Autodesk Inventor part; units mm, degrees
ref_plane "YZ Plane" through (0, 0, 0) normal (1, 0, 0) x (0, 1, 0)
ref_plane "XZ Plane" through (0, 0, 0) normal (0, 1, 0) x (-1, 0, 0)
ref_plane "XY Plane" through (0, 0, 0) normal (0, 0, 1) x (1, 0, 0)
sketch "Sketch1" plane through (0, 0, 0) normal (0, 1, 0) x (-1, 0, 0)
  line L0 (0, 0) -> (-37, 0)
  line L1 (-37, 0) -> (-37, 37)
  line L2 (-37, 37) -> (0, 37)
  line L3 (0, 37) -> (0, 0)
  circle A0 centre (-18.5, 18.5) radius 15.5
  point P0 (-18.5, 0)
  dimension "d0" = 37
  dimension "d1" = 37
  dimension "d2" = 18.5
  dimension "d3" = 18.5
  dimension "d4" = 31
extrude "Extrusion1" add sketch "Sketch1" against normal blind 35
sketch "Sketch3" plane through (0, 0, 37) normal (0, 0, 1) x (1, 0, 0)
  circle A0 centre (18.5, -10) radius 4.5
  line L0 (37, 0) -> (37, -35)
  point P0 (0, 0)
  dimension "d8" = 9
  dimension "d18" = 18.5
extrude "Extrusion2" cut sketch "Sketch3" against normal blind 5
sketch "Sketch4" plane through (37, 0, 0) normal (0, 0, -1) x (-1, 0, 0)
  circle A0 centre (18.5, -10) radius 4.5
  circle A1 centre (18.5, -10) radius 2.5
  point P0 (37, 0)
  dimension "d11" = 5
extrude "Extrusion3" cut sketch "Sketch4" against normal blind 5 contours A1
sketch "Sketch5" plane through (0, 0, 37) normal (0, 0, 1) x (1, 0, 0)
  line L0 (37, 0) -> (0, 0)
  line L1 (0, -35) -> (37, -35)
  line L2 (0, 0) -> (37, 0)
  line L3 (37, 0) -> (37, -35)
  line L4 (37, -35) -> (0, -35)
  line L5 (0, -35) -> (0, 0)
  line L6 (0, 0) -> (0, -35)
  line L7 (0, 0) -> (37, 0)
  line L8 (37, 0) -> (37, -35)
  line L9 (37, -35) -> (0, -35)
  line L10 (0, -35) -> (0, 0)
  circle A0 centre (18.5, -25) radius 4.5
  dimension "d19" = 18.5
  dimension "d22" = 10
extrude "Extrusion4" add sketch "Sketch5" along normal blind 2
sketch "Sketch6" plane through (0, 0, 39) normal (0, 0, 1) x (1, 0, 0)
  line L0 (0, 0) -> (0, -35)
  line L1 (0, -35) -> (37, -35)
  line L2 (0, 0) -> (37, 0)
  line L3 (37, 0) -> (37, -35)
  line L4 (37, -35) -> (0, -35)
  line L5 (0, -35) -> (0, 0)
extrude "Extrusion5" add sketch "Sketch6" along normal blind 5
sketch "Sketch7" plane through (0, 0, 44) normal (0, 0, 1) x (1, 0, 0)
  circle A0 centre (18.5, -10) radius 2.5
  line L0 (37, 0) -> (0, 0)
  line L1 (37, -35) -> (37, 0)
  point P0 (18.5, 0)
  dimension "d24" = 5
  dimension "d25" = 10
  dimension "d26" = 18.5
extrude "Extrusion6" cut sketch "Sketch7" against normal through all
equation "\"d0\" = d1"
properties part number "welco mount v03b"
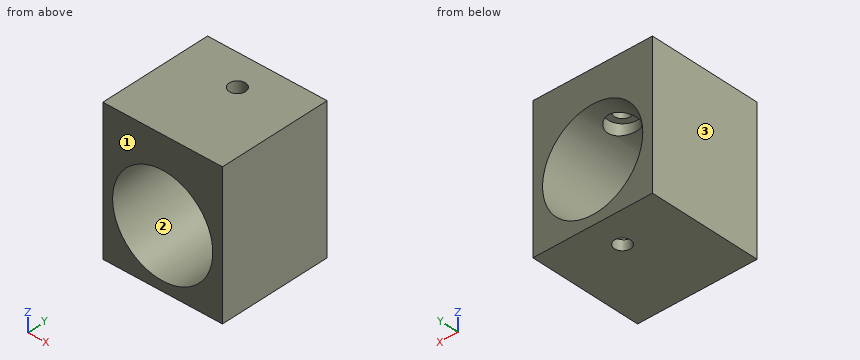
CAD build for the part. Positions are in the model's coordinates, mm. Face numbers are marked on the shaded views. Coordinates: 2 decimals unless noted, no trailing zeros. Loops run counter-clockwise (first coordinate to the right, second up) from the corner with the lowest first, then second, coordinate; pieces in that order, holes last. Notation, with made-up numbers: (19, -7.5) - (26, -7.5) arc R26 cw to (26, 7.5) - close; hole circle Ø9 at (-38, -13). An arc over 180 degrees is marked (long way). Use CSV: the item, a comma, the result in double quotes. Start each with the question number.
Q1. Cut at D-D, the plane x = 31.5. List the corners of the cut face in (y, z), then the cut area to 3 significant figures.
Q2. Cut at B-B, the plane z = 18.5. List the corners of the cut face in (x, y), then the cut area to 3 significant figures.
Q3. Two-plate mould, pull along X, no slides. Class the marked faces 1, 2 and 3: +X half, -X half, draft (parallel to the pull), parting line (faces both ways), or undercut.
Q4. Cut at C-C, the plane y = -10. List the corners of the cut face in (x, z).
Q5. Cut at A-A, the plane x = 18.5. List the corners of the cut face in (y, z).
Q6. Probe probe 1 along Z at (x, y) = (18, -21); probe 2 along Y at (x, z) = (18, 38); probe 3 along Z at (x, y) = (18.5, -0.5). List the from-to ranges inside material, lowest first. Write a range as from..to.
Here are the results:
1,outline,"(-35, 0) - (0, 0) - (0, 10.06) - (-35, 10.06) - close; (-35, 26.94) - (0, 26.94) - (0, 44) - (-35, 44) - close"
1,area,"949 mm2"
2,outline,"(0, -35) - (3, -35) - (3, 0) - (0, 0) - close; (34, -35) - (37, -35) - (37, 0) - (34, 0) - close"
2,area,"210 mm2"
3,face 1,"draft"
3,face 2,"undercut"
3,face 3,"-X half"
4,outline,"(0, 0) - (16, 0) - (16, 3.2) arc R15.5 cw to (14, 33.33) - (14, 37) - (16, 37) - (16, 44) - (0, 44) - close; (21, 0) - (37, 0) - (37, 44) - (21, 44) - (21, 37) - (23, 37) - (23, 33.33) arc R15.5 cw to (21, 3.2) - close"
5,outline,"(-35, 0) - (-12.5, 0) - (-12.5, 3) - (-35, 3) - close; (-35, 34) - (-14.5, 34) - (-14.5, 37) - (-12.5, 37) - (-12.5, 44) - (-35, 44) - close; (-7.5, 0) - (0, 0) - (0, 3) - (-7.5, 3) - close; (-7.5, 37) - (-5.5, 37) - (-5.5, 34) - (0, 34) - (0, 44) - (-7.5, 44) - close; hole (-29.5, 37) - (-20.5, 37) - (-20.5, 39) - (-29.5, 39) - close"
6,probe 1,"0..3.01, 33.99..37, 39..44"
6,probe 2,"-35..-29.47, -20.53..-12.45, -7.55..0"
6,probe 3,"0..3, 34..44"
